from build123d import *

# Parameters (mm, degrees)
SKETCH1_R           = 11.5
SKETCH1_R_2         = 8.0883
BOSS_EXTRUDE1_DEPTH = 36.88
CUT_EXTRUDE1_DEPTH  = 55.88
SKETCH3_R           = 1.075360457
CUT_EXTRUDE2_DEPTH  = 41.306753925


with BuildPart() as part:
    # Sketch1 → Boss-Extrude1 (new body)
    with BuildSketch(Plane(origin=(0, 0, 0), x_dir=(1, 0, 0), z_dir=(0, 1, 0))):
        with Locations(Location((0, 0, 0), (0, 0, 270))):
            Circle(SKETCH1_R)
        with Locations(Location((0, 0, 0), (0, 0, 270))):
            Circle(SKETCH1_R_2, mode=Mode.SUBTRACT)
    extrude(amount=BOSS_EXTRUDE1_DEPTH)

    # Sketch2 → Cut-Extrude1 (cut)
    with BuildSketch(Plane.ZY.offset(11.5)):
        with BuildLine():
            Line((3.302, 32.573327327), (3.302, 4.306672673))
            ThreePointArc((3.302, 4.306672673), (0, 1.004672673), (-3.302, 4.306672673))
            Line((-3.302, 4.306672673), (-3.302, 32.573327327))
            ThreePointArc((-3.302, 32.573327327), (0, 35.875327327), (3.302, 32.573327327))
        make_face()
    extrude(amount=-CUT_EXTRUDE1_DEPTH, mode=Mode.SUBTRACT)

    # Sketch3 → Cut-Extrude2 (cut, through all)
    with BuildSketch(Plane.XY):
        with Locations(Location((0, 18.44, 0), (0, 0, 270.000000024))):
            Circle(SKETCH3_R)
    extrude(amount=CUT_EXTRUDE2_DEPTH, mode=Mode.SUBTRACT)


solid = part.part
Can you work these out from the model? Positions are in its coordinate system, mm. A direction names the side the tool comes from. Coordinates: 2 decimals unless noted, no trailing zeros. Loops run counter-clockwise (first coordinate to the right, second up) from the corner with the lowest first, then second, coordinate; pieces in that order, holes last. Notation, with made-up numbers: (40.5, -11.5) - (75.5, -11.5) arc R28 ccw to (75.5, 26.5) - close; hole circle Ø3 at (-37, 61). An arc over 180 degrees is marked (long way). Answer as a JSON object with one key per item and string values. Group by question number.
Item 1: If we section it at A-A (z = 0): List the corners of the cut face in (x, y) for me, plus the area to 3 significant figures.
Item 2: If we section it at B-B (y = 22.5): List the corners of the cut face in (x, z) for me.
Item 3: For pin 1 (2 mm diameter, centred on x = 3, y = 5.5, fed in from -Z); pin 2 (1.1 mm diameter, centred on x = -9.5, y = 17.5, fed in from +Z); pin 3 (1.5 mm diameter, centred on y = 16, z = -5.5, fed in from +X), each with a flat end and sliding along its axis, tell me the tip position at first contact or that it passes through.
Item 4: If we mould it in two halves opening along Y, with no side actions, what happens to faces 4 (the face through (8, 36.88, 2)), 5 (the face through (8, 0, 2)), 6 (the face through (-9.471, 1.005, 0.073))? For each: released by +Y, released by -Y, zero draft, split by the parting line, or undercut.
Item 5: If we section it at C-C (x = 0): List the corners of the cut face in (y, z) for me, plus the area to 3 significant figures.
Item 6: If I drill on L1, parallel to Z at x = 7.25, y = 11; L2, parallel to Z at x = 2.5, y = 20; L3, parallel to X at y = 18.44, z = 9.15, over which ranges is the centre line in solid material (lowest first)? Write a range as from..to.
Item 7: On a 3-axis mill with a long thin cutter (end or side, diameter ignored), from which of +Z, -Z, +X, -X, +Y, -Y can I reach the whole of each face in a straight line? I mean faces 1 (the face through (0.323, 17.414, 9.734)), 2 (the face through (-9, 18, -3.302)), 3 (the face through (-4.405, 18.182, 10.623)). Say none if no direction works.
Item 8: If we section it at D-D (y = 18.44): List the corners of the cut face in (x, z) for me, plus the area to 3 significant figures.
Returned:
{
 "1": {"outline": "(-11.5, 0) - (-8.09, 0) - (-8.09, 1) - (-11.5, 1) - close; (-11.5, 35.88) - (-8.09, 35.88) - (-8.09, 36.88) - (-11.5, 36.88) - close; (8.09, 0) - (11.5, 0) - (11.5, 1) - (8.09, 1) - close; (8.09, 35.88) - (11.5, 35.88) - (11.5, 36.88) - (8.09, 36.88) - close", "area": "13.7 mm²"},
 "2": {"outline": "(-11.02, -3.3) arc R11.5 ccw to (11.02, -3.3) - (7.38, -3.3) arc R8.09 cw to (-7.38, -3.3) - close; (-11.02, 3.3) - (-7.38, 3.3) arc R8.09 cw to (7.38, 3.3) - (11.02, 3.3) arc R11.5 ccw to start"},
 "3": {"pin 1": "stops at z = -11.32", "pin 2": "stops at z = 7.22", "pin 3": "stops at x = 10.47"},
 "4": {"face 4": "released by +Y", "face 5": "released by -Y", "face 6": "undercut"},
 "5": {"outline": "(0, -11.5) - (36.88, -11.5) - (36.88, -8.09) - (0, -8.09) - close; (0, 8.09) - (17.36, 8.09) - (17.36, 11.5) - (0, 11.5) - close; (19.52, 8.09) - (36.88, 8.09) - (36.88, 11.5) - (19.52, 11.5) - close", "area": "244 mm²"},
 "6": {"L1": "z = -8.93..-3.59, 3.59..8.93", "L2": "z = -11.22..-7.69, 7.69..11.22", "L3": "x = -6.97..-1.08, 1.08..6.97"},
 "7": {"face 1": "+Z", "face 2": "+X, -X", "face 3": "+Y, -Y"},
 "8": {"outline": "(-11.02, -3.3) arc R11.5 ccw to (11.02, -3.3) - (7.38, -3.3) arc R8.09 cw to (-7.38, -3.3) - close; (-11.02, 3.3) - (-7.38, 3.3) arc R8.09 cw to (-1.08, 8.02) - (-1.08, 11.45) arc R11.5 ccw to start; (1.08, 8.02) arc R8.09 cw to (7.38, 3.3) - (11.02, 3.3) arc R11.5 ccw to (1.08, 11.45) - close", "area": "157 mm²"}
}
